from build123d import *

# Parameters (mm, degrees)
F1_DEPTH = 10
F2_R     = 10


with BuildPart() as f1:
    # F0 (on Top) → F1 (new body)
    with BuildSketch(Plane.XY):
        Polygon((40.5, 60), (25.5, 60), (25.5, 0), (0, 0), (-25.5, 0), (-25.5, 60), (-40.5, 60), (-40.5, -45.930237), (-20, -45.930237), (-20, -145.930237), (0, -145.930237), (20, -145.930237), (20, -45.930237), (40.5, -45.930237), align=None)
    extrude(amount=F1_DEPTH)

    # F2
    f2_edges = [f1.edges().sort_by_distance(p)[0] for p in [
        (20, -145.930237, 5),
        (-20, -145.930237, 5),
        (40.5, -45.930237, 5),
        (20, -45.930237, 5),
        (-40.5, -45.930237, 5),
        (-20, -45.930237, 5),
        (25.5, 0, 5),
        (-25.5, 0, 5),
        (40.5, 60, 5),
        (-40.5, 60, 5),
    ]]
    fillet(f2_edges, radius=F2_R)


solid = f1.part
Verification items for the finished model (mm, model axes). A direction names the side the tool comes from. Give positions to 0.01 mm unless a question says otherwise; leave off trailing zeros. Write each loop counter-clockwise with the first axis right and the second up, starting at its lowest first coordinate (ties: lowest second). Pieces come first, ordered by that corner, then holes.
(1) Material ranges on line 1 (X direction, y = 30.5, z = 8.5); line 2 (X direction, y = -132, z = 3.25); line 3 (Y direction, x = -7, z = 8.5), recorded low to high.
(2) Gauge pin test, flat ends, axial feed: pin 1 (6 mm diameter, centred on x = 10.5, z = 1.5, fed in from +Y); pin 2 (4 mm diameter, centred on y = -82, z = 5, fed in from +X); pin 3 (4 mm diameter, centred on x = 27, z = 7, fed in from -Y). Record the tip position at first contact, or that the pin passes through.
(3) Cross-section at B-B (z = 7). Enter the section's corners in (x, y).
(4) Cross-section at A-A (y = 17). Enter the section's corners in (x, z), plus the area to 3 significant figures.
(5) Cross-section at C-C (x = 7.5). Enter the section's corners in (y, z).
(6) Cross-section at D-D (y = -66.5). Enter the section's corners in (x, z).
(7) Access from +Z, -Z, +X, -X, +Y, -Y to the whole of each face (thin tool, end or side, straight path). Record for faces 1 (the face through (-28, 60, 5)), 2 (the face through (-20, -95, 5)), 3 (the face through (-40.5, 8, 5)), 4 (the face through (20, -96, 5)), 5 (the face through (0, 0, 5)).
(8) Mould release check, pull along Z, two halves, no side actions. Record for faces 6 (the face through (40.5, 6, 5)), 7 (the face through (-1, -42, 10)), 8 (the face through (-1, -42, 0)): +Z half, -Z half, draft (parallel to the pull), parting line (faces both ways), or undercut.
Worked out:
1. line 1: x = -40.5 to -25.5, 25.5 to 40.5
1. line 2: x = -20 to 20
1. line 3: y = -145.93 to 0
2. pin 1: stops at y = 0
2. pin 2: stops at x = 20
2. pin 3: stops at y = -47.27
3. outline: (-40.5, -35.93) arc R10 ccw to (-30.5, -45.93) - (-30, -45.93) arc R10 cw to (-20, -55.93) - (-20, -135.93) arc R10 ccw to (-10, -145.93) - (10, -145.93) arc R10 ccw to (20, -135.93) - (20, -55.93) arc R10 cw to (30, -45.93) - (30.5, -45.93) arc R10 ccw to (40.5, -35.93) - (40.5, 50) arc R10 ccw to (30.5, 60) - (25.5, 60) - (25.5, 10) arc R10 cw to (15.5, 0) - (-15.5, 0) arc R10 cw to (-25.5, 10) - (-25.5, 60) - (-30.5, 60) arc R10 ccw to (-40.5, 50) - close
4. outline: (-40.5, 0) - (-25.5, 0) - (-25.5, 10) - (-40.5, 10) - close; (25.5, 0) - (40.5, 0) - (40.5, 10) - (25.5, 10) - close
4. area: 300 mm2
5. outline: (-145.93, 0) - (0, 0) - (0, 10) - (-145.93, 10) - close
6. outline: (-20, 0) - (20, 0) - (20, 10) - (-20, 10) - close
7. face 1: +Z, -Z, +X, -X, +Y
7. face 2: +Z, -Z, -X, -Y
7. face 3: +Z, -Z, -X, +Y, -Y
7. face 4: +Z, -Z, +X, -Y
7. face 5: +Z, -Z, +Y
8. face 6: draft
8. face 7: +Z half
8. face 8: -Z half
